Source: three-view drawing plus pictorial views. Frame: mm from the lowest corner of the part. A direction names the side the tool comes from. Give positions to 0.01 mm unless a question says otherwise; leave off trailing zeros. Write each loop counter-clockwise with the first axis right and the second up, starting at its lowest first coordinate (ties: lowest second). Pieces come first, ordered by that corner, then holes.
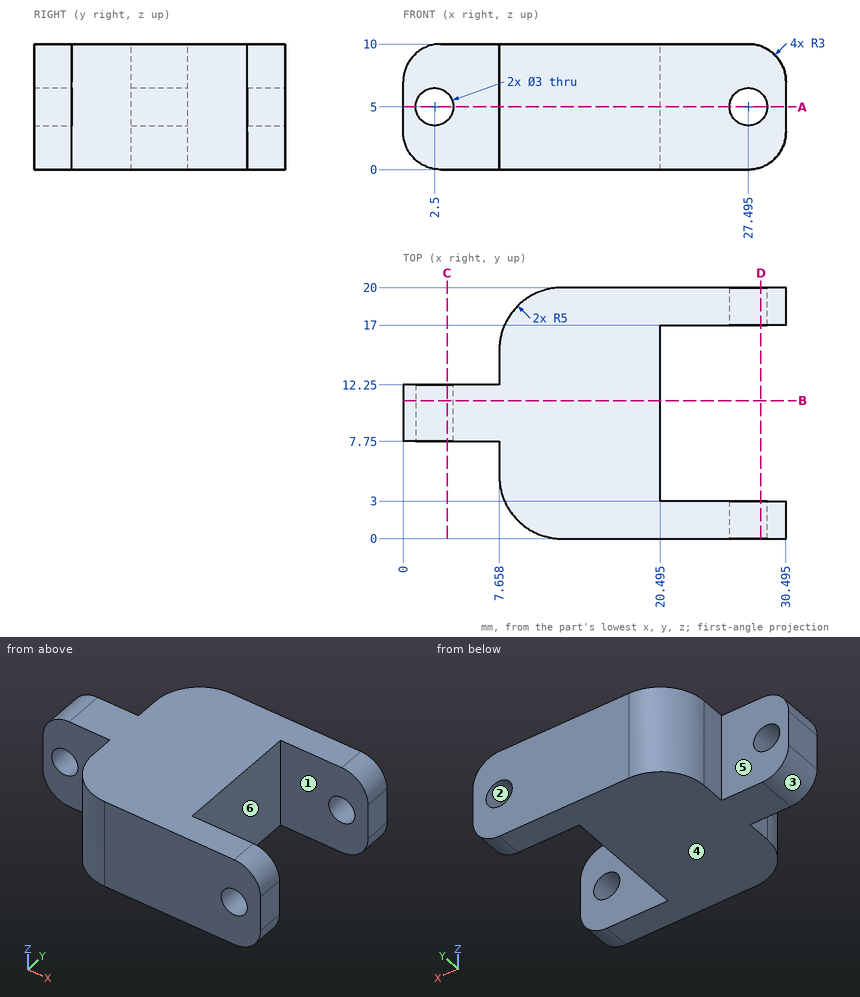
Q1. Section B-B on y = 11. Output: boundary loops of the cut face in (x, z) (1 decimal).
Filled sheet:
outline: (0, 3) arc R3 ccw to (3, 0) - (20.5, 0) - (20.5, 10) - (3, 10) arc R3 ccw to (0, 7) - close; hole circle Ø3 at (2.5, 5)
Q2. Ray query, line 1 along Y through (x, z) = (27, 2); line 2 along Z through (x, y) = (2.5, 10.2); line 3 along X through (y, z) = (12.5, 4.5) (1 decimal). Return the intervals inside material, ascending.
Filled sheet:
line 1: y = 0 to 3, 17 to 20
line 2: z = 0.04 to 3.5, 6.5 to 9.96
line 3: x = 7.7 to 20.5
Q3. Section A-A on z = 5. Count the separate pieces of the cut face and the enclosed holes in it, plus the area to 3 significant figures.
Filled sheet:
separate pieces: 4
enclosed holes: 0
area: 309 mm2
Q4. Section D-D on x = 28.5. Output: boundary loops of the cut face in (y, z).
Filled sheet:
outline: (0, 0.17) - (3, 0.17) - (3, 3.89) - (0, 3.89) - close; (0, 6.11) - (3, 6.11) - (3, 9.83) - (0, 9.83) - close; (17, 0.17) - (20, 0.17) - (20, 3.89) - (17, 3.89) - close; (17, 6.11) - (20, 6.11) - (20, 9.83) - (17, 9.83) - close
Q5. Access query for the marked faces 4, 5 and 6. Directions: +Z, -Z, +X, -X, +Y, -Y. A direction counts if a zero-diameter tool reaches every point of the face in a straight line with its end or side. Return the directions, or none.
Filled sheet:
face 4: -Z, +X, -X, +Y, -Y
face 5: +Z, -Z, -X, +Y
face 6: +Z, -Z, +X
Q6. Pin query (flat end, axial travel): P1, Ø1.4, axis at y = 6.5, z = 7.5, coming from the -X side; P2, Ø1.5, axis at y = 10, z = 7, coming from the -X side; P3, Ø2.5, axis at x = 4, z = 4.5, coming from the +Y side. Return the tip coordinate at first contact, or that it passes through.
Filled sheet:
P1: stops at x = 7.66
P2: stops at x = 0
P3: stops at y = 12.25
Q7. Section C-C on x = 3.5. Output: boundary loops of the cut face in (y, z).
Filled sheet:
outline: (7.75, 0) - (12.25, 0) - (12.25, 3.88) - (7.75, 3.88) - close; (7.75, 6.12) - (12.25, 6.12) - (12.25, 10) - (7.75, 10) - close
Q8. Pull-direction query (X, two-part tool) for the marked faces 1, 2 and 3; classes: released by +X, released by -X, zero draft, split by the parting line, or undercut.
Filled sheet:
face 1: zero draft
face 2: undercut
face 3: released by -X
